```python
from build123d import *

# Parameters (mm, degrees)
CUT_EXTRUDE1_START = -3.175
CUT_EXTRUDE1_DEPTH = 6.35


with BuildPart() as part:
    # Sketch1 → Revolve1 (revolve)
    with BuildSketch(Plane.XY):
        Polygon((369.442161905, 123.802816275), (567.864710706, 27.346117543), (567.14289772, 25.861265021), (368.720348919, 122.317963753), align=None)
    revolve(axis=Axis((549.918417615, 44.825187693, 0), (0.89936555, -0.437197448, 0)))

    # Sketch2 → Cut-Extrude1 (cut)
    with BuildSketch(Plane.XY.offset(CUT_EXTRUDE1_START)):
        Polygon((552.627624135, 54.098993909), (575.471509095, 42.994178741), (567.14289772, 25.861265021), (544.299012759, 36.966080188), align=None)
    extrude(amount=CUT_EXTRUDE1_DEPTH, mode=Mode.SUBTRACT)


solid = part.part
```
CAD build for the part. Positions are in the model's coordinates, mm. Round coordinates to 2 decimals unless told otherwise and drop trailing zeros. Order: outer loops, then holes, each group sorted by start corner. A loop starts at its lowest first (then second) coordinate and runs counter-clockwise, first axis right, second up. Notation, with made-up numbers: (-6.5, 40.5) - (36.5, 40.5) arc R20 ccw to (36.5, 45.5) - close; hole circle Ø4 at (16, 0). An arc over 180 degrees is marked (long way). Use CSV: the item, a comma, the result in double quotes. Start each with the question number.
1) Wall check: L1, parallel to Z at x = 526, y = 57; L2, parallel to Y at x = 393.5, z = -5.5; L3, parallel to Z at x = 486.5, y = 83.5. Give the ranges that are in metal, low to high. Write a range as [from, to].
2) Pin check, flat tips, straight feed: pin 1 Ø1 at (x, z) = (392.5, 2.5) entering from -Y; pin 2 Ø4 at (x, y) = (564.5, 46.5) entering from -Z; pin 3 Ø6.5 at (x, y) = (564, 46.5) entering from +Z. Stop position of each tip, or through.
3) Saw through at A-A (z = -5.75). List the corners of the cut face in (x, y).
4) Two-plate mould, pull along Y, no slides. Class faces 1 (the cylindrical face through (476.924, 89.056, -0.346)), 2 (the flat face through (563, 47, -3.175)), 3 (the cylindrical face through (468.79, 79.38, 8.45)), 4 (the flat face through (571.58, 34.99, -8.01)): pulls with the +Y half, pulls with the -Y half, needs draft (parallel to the pull), parting line crosses it, or undercut.
Values follow:
1,L1,"z = [-9.51, -7.86], [7.86, 9.51]"
1,L2,"y = [112.22, 114.6], [127.13, 129.51]"
1,L3,"z = [-6.4, -3.49], [3.49, 6.4]"
2,pin 1,"stops at y = 110.85"
2,pin 2,"stops at z = -7.49"
2,pin 3,"stops at z = 8.44"
3,outline,"(369.56, 124.05) - (567.99, 27.6) - (568.96, 29.59) - (370.53, 126.05) - close; (375.24, 135.72) - (573.66, 39.27) - (574.63, 41.26) - (376.2, 137.71) - close"
4,face 1,"undercut"
4,face 2,"needs draft"
4,face 3,"parting line crosses it"
4,face 4,"pulls with the -Y half"
